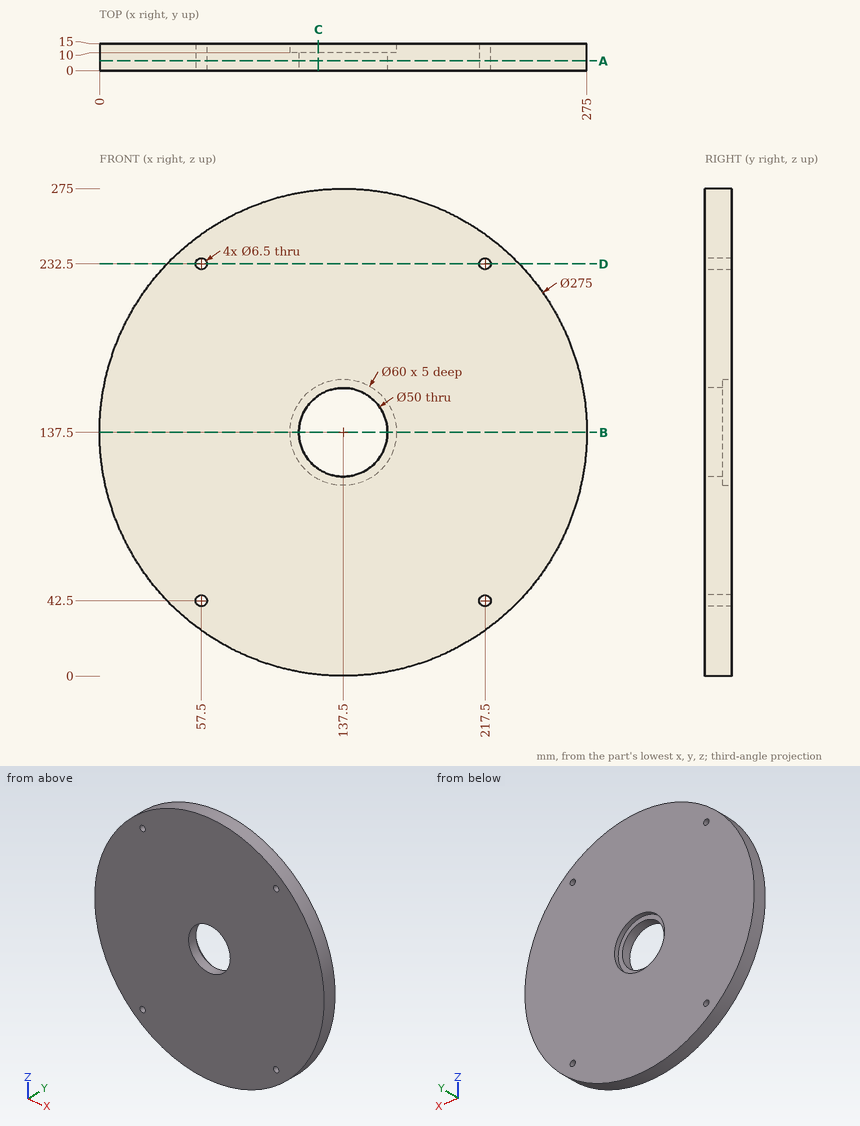
Here's the drawing with two shaded views (mm, measured from the low corner). I have some questions. Coordinates: 2 decimals unless noted, no trailing zeros. Order: outer loops, then holes, each group sorted by start corner. A loop starts at its lowest first (then second) coordinate and runs counter-clockwise, first axis right, second up.
Item 1: For P1, Ø6, axis at x = 159.5, y = 3, coming from the +Z side; P2, Ø3, axis at y = 5, z = 94, coming from the +X side; P3, Ø2, axis at x = 34.5, y = 6.5, coming from the +Z side, each with a flat end and sliding along its axis, tell me the tip position at first contact or that it passes through.
Result sheet:
P1: stops at z = 273.68
P2: stops at x = 268.43
P3: stops at z = 229.71
Item 2: If we section it at C-C on x = 123.5: List the corners of the cut face in (y, z) for me, plus the area to 3 significant figures.
Result sheet:
outline: (0, 0.71) - (15, 0.71) - (15, 110.97) - (10, 110.97) - (10, 116.79) - (0, 116.79) - close; (0, 158.21) - (10, 158.21) - (10, 164.03) - (15, 164.03) - (15, 274.29) - (0, 274.29) - close
area: 3,420 mm2
Item 3: If we section it at A-A on y = 5.5: List the corners of the cut face in (x, z) for me, plus the area to 3 significant figures.
Result sheet:
outline: circle Ø275 at (137.5, 137.5); hole circle Ø6.5 at (57.5, 42.5); hole circle Ø6.5 at (57.5, 232.5); hole circle Ø50 at (137.5, 137.5); hole circle Ø6.5 at (217.5, 42.5); hole circle Ø6.5 at (217.5, 232.5)
area: 57,300 mm2
Item 4: I need wall thicknesses on line 1 (Z direction, x = 217.5, y = 8.5); line 2 (Z direction, x = 137.5, y = 13.8). Which ranges of each line are inside material? Lowest first, please.
Result sheet:
line 1: z = 25.67 to 39.25, 45.75 to 229.25, 235.75 to 249.33
line 2: z = 0 to 107.5, 167.5 to 275
Item 5: If we section it at D-D on z = 232.5: List the corners of the cut face in (x, y) for me, plus the area to 3 significant figures.
Result sheet:
outline: (38.1, 0) - (54.25, 0) - (54.25, 15) - (38.1, 15) - close; (60.75, 0) - (214.25, 0) - (214.25, 15) - (60.75, 15) - close; (220.75, 0) - (236.9, 0) - (236.9, 15) - (220.75, 15) - close
area: 2,790 mm2
Item 6: If we section it at B-B on z = 137.5: List the corners of the cut face in (x, y) for me.
Result sheet:
outline: (0, 0) - (112.5, 0) - (112.5, 10) - (107.5, 10) - (107.5, 15) - (0, 15) - close; (162.5, 0) - (275, 0) - (275, 15) - (167.5, 15) - (167.5, 10) - (162.5, 10) - close
